Geometry: final body of the model. Coordinates: model frame, mm. A direction names the side the tool comes from. Round coordinates to 2 decimals unless told otherwise and drop trailing zeros. Loops run counter-clockwise (first coordinate to the right, second up) from the corner with the lowest first, then second, coordinate; pieces in that order, holes last. Notation, with made-up numbers: (15.25, 17.5) - (42.25, 17.5) arc R33 ccw to (42.25, 50.5) - close; hole circle Ø4 at (18.25, 7). An arc over 180 degrees is marked (long way). Answer as a JSON object with one key per item and string values. Group by question number.
Item 1: Line query: line 1 (X direction, y = -27, z = 23); line 2 (Y direction, x = -9.5, z = 10); line 3 (Z direction, x = -4, y = -50.5). Output: solid intervals per line, ascending.
Item 2: Section C-C (x = 18). Return the cut outline in (y, z).
Item 3: Section B-B (y = 47). Return the cut outline in (x, z).
Item 4: Reachability of faces 1 (the face through (48.861, -83.293, 23.72)), 2 (the face through (-1, -100, 22)) from +Z, -Z, +X, -X, +Y, -Y: full face, straight path, thin tool, end or side. Return the list, or none.
Item 5: Section A-A (z = 17). Return the cut outline in (x, y).
Item 6: Draft query along X for faces 3 (the face through (-57, 1, 24)), 4 (the face through (60, -1, 22)), 5 (the face through (-51.46, -84.79, 21.69)). Return one class per face: released by +X, released by -X, zero draft, split by the parting line, or undercut.
Item 7: First-contact query: pin 1 (4 mm diameter, centred on x = -13, y = 31, fed in from +Z); pin 2 (12 mm diameter, centred on x = -28, y = -41, fed in from -Z). Flat tips, straight axial feed; report the tip coordinate or a pass-through.
```python
from build123d import *

# Parameters (mm, degrees)
BOSS_EXTRUDE1_DEPTH = 4
BOSS_EXTRUDE2_DEPTH = 40


with BuildPart() as part:
    # Sketch1 → Boss-Extrude1 (new body)
    with BuildSketch(Plane.XY):
        Polygon((-60, 70), (-26.436014753, 110), (26.436014753, 110), (60, 70), (60, -70), (42.679491924, -100), (-42.679491924, -100), (-60, -70), align=None)
    extrude(amount=BOSS_EXTRUDE1_DEPTH)

    # Sketch2 → Boss-Extrude2 (add)
    with BuildSketch(Plane.XY.offset(4)):
        Polygon((-26.436014753, 110), (-60, 70), (-60, -70), (-42.679491924, -100), (42.679491924, -100), (60, -70), (60, 70), (26.436014753, 110), align=None)
        Polygon((-25.037091778, 107), (-57, 68.908089297), (-57, -69.196152423), (-40.947441117, -97), (40.947441117, -97), (57, -69.196152423), (57, 68.908089297), (25.037091778, 107), align=None, mode=Mode.SUBTRACT)
    extrude(amount=BOSS_EXTRUDE2_DEPTH)


solid = part.part
```
Values:
{
 "1": {"line 1": "x = -60 to -57, 57 to 60", "line 2": "y = -100 to -97, 107 to 110", "line 3": "z = 0 to 4"},
 "2": {"outline": "(-100, 0) - (110, 0) - (110, 44) - (107, 44) - (107, 4) - (-97, 4) - (-97, 44) - (-100, 44) - close"},
 "3": {"outline": "(-60, 0) - (60, 0) - (60, 44) - (57, 44) - (57, 4) - (-57, 4) - (-57, 44) - (-60, 44) - close"},
 "4": {"face 1": "+Z", "face 2": "+Z, -Z, +X, -X, -Y"},
 "5": {"outline": "(-60, -70) - (-42.68, -100) - (42.68, -100) - (60, -70) - (60, 70) - (26.44, 110) - (-26.44, 110) - (-60, 70) - close; hole (-57, -69.2) - (-40.95, -97) - (40.95, -97) - (57, -69.2) - (57, 68.91) - (25.04, 107) - (-25.04, 107) - (-57, 68.91) - close"},
 "6": {"face 3": "undercut", "face 4": "released by +X", "face 5": "released by -X"},
 "7": {"pin 1": "stops at z = 4", "pin 2": "stops at z = 0"}
}
